Geometry check sheet. Reference: the model listing, model coordinates, mm. Round coordinates to 2 decimals unless told otherwise and drop trailing zeros. Order: outer loops, then holes, each group sorted by start corner. A loop starts at its lowest first (then second) coordinate and runs counter-clockwise, first axis right, second up. Notation, with made-up numbers: (-13.5, 58.5) -> (44.5, 58.5) arc R26 cw to (44.5, 88.5) -> close; hole circle Ø4 at (89.25, 24). An arc over 180 degrees is marked (long way). Answer as a JSON object with one key per item and string values. Group by question number.
from build123d import *

# Parameters (mm, degrees)
BASPROSKE_W         = 3
BASPROSKE_H         = 7
TOOTHCUT_DEPTH      = 11.344080433
TEETHCUTS_COUNT     = 12
BORSKE_R            = 2.9
BORE_DEPTH          = 50.0000508
CUT_EXTRUDE_1_DEPTH = 1.5


with BuildPart() as part:
    # BasProSke → Base-Revolve (revolve)
    with BuildSketch(Plane(origin=(0, 0, 0), x_dir=(1, 0, 0), z_dir=(0, 1, 0)), mode=Mode.PRIVATE) as base_revolve_sk:
        with Locations((1.5, 3.5)):
            Rectangle(BASPROSKE_W, BASPROSKE_H)
    revolve(base_revolve_sk.sketch.rotate(Axis((-10, 0, 0), (1, 0, 0)), 180), axis=Axis((-10, 0, 0), (1, 0, 0)))

    # TooCutSke → ToothCut (cut, through all)
    with BuildSketch(Plane(origin=(0, 0, 0), x_dir=(0, 0, -1), z_dir=(1, 0, 0))):
        with BuildLine():
            ThreePointArc((0.562207301, 4.715604304), (0, 4.749), (-0.562207301, 4.715604304))
            ThreePointArc((-0.562207301, 4.715604304), (-0.837528627, 5.917009812), (-1.672850686, 6.823328788))
            ThreePointArc((-1.672850686, 6.823328788), (0, 7.0254), (1.672850686, 6.823328788))
            ThreePointArc((1.672850686, 6.823328788), (0.837528627, 5.917009812), (0.562207301, 4.715604304))
        make_face()
    toothcut = extrude(amount=TOOTHCUT_DEPTH, mode=Mode.SUBTRACT)

    # TeethCuts: ToothCut ×12 about axis
    teethcuts_axis = Axis((0, 0, 0), (1, 0, 0))
    for i in range(1, TEETHCUTS_COUNT):
        add(toothcut.rotate(teethcuts_axis, i * 360 / TEETHCUTS_COUNT), mode=Mode.SUBTRACT)

    # BorSke → Bore (cut, symmetric)
    with BuildSketch(Plane(origin=(0, 0, 0), x_dir=(0, 0, -1), z_dir=(1, 0, 0))):
        with Locations(Location((0, 0, 0), (0, 0, 180))):
            Circle(BORSKE_R)
    extrude(amount=BORE_DEPTH, both=True, mode=Mode.SUBTRACT)

    # 草图1 → 切除-拉伸1 (cut)
    with BuildSketch(Plane(origin=(3, 0, 0), x_dir=(0, 0, -1), z_dir=(1, 0, 0))):
        Polygon((-1.6, -1.6), (-1.6, -3.5), (1.6, -3.5), (1.6, -1.6), (3.5, -1.6), (3.5, 1.6), (1.6, 1.6), (1.6, 3.5), (-1.6, 3.5), (-1.6, 1.6), (-3.5, 1.6), (-3.5, -1.6), align=None)
    extrude(amount=-CUT_EXTRUDE_1_DEPTH, mode=Mode.SUBTRACT)


solid = part.part
Item 1: Mould release check, pull along Z, two halves, no side actions. Record for faces 1 (the cylindrical face through (1.479, -2.233, 5.543)), 2 (the flat face through (2, -3, 1.6)): pulls with the +Z half, pulls with the -Z half, needs draft (parallel to the pull), parting line crosses it, or undercut.
Item 2: Sectioned sample at C-C, the plane y = -4. Enter the section's corners in (x, z), then the cut area to 3 significant figures.
Item 3: Thickness scan on L1, parallel to Z at x = 1.8, y = 4.25; L2, parallel to Z at x = 2.3, y = 0; L3, parallel to Y at x = 2.25, z = 4. Record the ranges inside material, lowest first.
Item 4: Sectioned sample at A-A, the plane y = 0. Enter the section's corners in (x, z).
Item 5: Depth check by flat-ended pin: pin 1 Ø0.9 at (x, z) = (2.5, 3) entering from -Y; pin 2 Ø0.5 at (x, z) = (2.5, -3) entering from +Y; pin 3 Ø0.9 at (x, y) = (2.5, 3) entering from -Z. Enter the tip coordinate at first touch or a pass-through.
Result:
{
 "1": {"face 1": "undercut", "face 2": "undercut"},
 "2": {"outline": "(0, -4.87) -> (3, -4.87) -> (3, -2.96) -> (0, -2.96) -> close; (0, -2.56) -> (3, -2.56) -> (3, 2.56) -> (0, 2.56) -> close; (0, 2.96) -> (3, 2.96) -> (3, 4.87) -> (0, 4.87) -> close", "area": "26.8 mm2"},
 "3": {"L1": "z = -4.97 to -3.15, -2.12 to 2.12, 3.15 to 4.97", "L2": "z = -4.75 to -3.5, 3.5 to 4.75", "L3": "y = -4.87 to -2.96, -2.56 to 2.56, 2.96 to 4.87"},
 "4": {"outline": "(0, -4.75) -> (3, -4.75) -> (3, -3.5) -> (1.5, -3.5) -> (1.5, -2.9) -> (0, -2.9) -> close; (0, 2.9) -> (1.5, 2.9) -> (1.5, 3.5) -> (3, 3.5) -> (3, 4.75) -> (0, 4.75) -> close"},
 "5": {"pin 1": "stops at y = -4.54", "pin 2": "stops at y = 4.36", "pin 3": "stops at z = -4.54"}
}
